```python
from build123d import *

# Parameters (mm, degrees)
F0_R      = 16.5
F17_DEPTH = 12
F18_DEPTH = 2


with BuildPart() as f17:
    # F0 (on Top) → F17 (new body)
    with BuildSketch(Plane.XY):
        with BuildLine():
            ThreePointArc((18.917614, -8.685167), (19.797247, -6.432516), (20.409685, -4.093046))
            ThreePointArc((20.409685, -4.093046), (20.714215, -2.056585), (20.816058, 0))
            ThreePointArc((20.816058, 0), (20.489002, 3.675464), (19.518114, 7.235432))
            ThreePointArc((19.518114, 7.235432), (18.547243, 9.450292), (17.326047, 11.537605))
            ThreePointArc((17.326047, 11.537605), (13.518948, 15.828654), (8.685167, 18.917614))
            ThreePointArc((8.685167, 18.917614), (6.432516, 19.797247), (4.093046, 20.409685))
            ThreePointArc((4.093046, 20.409685), (-1.633209, 20.751889), (-7.235432, 19.518114))
            ThreePointArc((-7.235432, 19.518114), (-9.450292, 18.547243), (-11.537605, 17.326047))
            ThreePointArc((-11.537605, 17.326047), (-15.828654, 13.518948), (-18.917614, 8.685167))
            ThreePointArc((-18.917614, 8.685167), (-19.797247, 6.432516), (-20.409685, 4.093046))
            ThreePointArc((-20.409685, 4.093046), (-20.751889, -1.633209), (-19.518114, -7.235432))
            ThreePointArc((-19.518114, -7.235432), (-18.547243, -9.450292), (-17.326047, -11.537605))
            ThreePointArc((-17.326047, -11.537605), (-13.518948, -15.828654), (-8.685167, -18.917614))
            ThreePointArc((-8.685167, -18.917614), (-6.432516, -19.797247), (-4.093046, -20.409685))
            ThreePointArc((-4.093046, -20.409685), (1.633209, -20.751889), (7.235432, -19.518114))
            ThreePointArc((7.235432, -19.518114), (9.450292, -18.547243), (11.537605, -17.326047))
            ThreePointArc((11.537605, -17.326047), (15.828654, -13.518948), (18.917614, -8.685167))
        make_face()
        Circle(F0_R, mode=Mode.SUBTRACT)
        with BuildLine():
            ThreePointArc((4.093046, 20.409685), (6.432516, 19.797247), (8.685167, 18.917614))
            Line((8.685167, 18.917614), (11.775337, 28.428179))
            Line((11.775337, 28.428179), (7.183216, 29.92025))
            Line((7.183216, 29.92025), (4.093046, 20.409685))
        make_face()
        Polygon((11.775337, 28.428179), (16.07751, 26.236113), (20.629834, 29.030011), (15.834552, 31.89982), (10.649371, 33.98415), (7.183216, 29.92025), align=None)
        Polygon((-16.07751, 26.236113), (-11.775337, 28.428179), (-7.183216, 29.92025), (-5.939822, 35.114813), (-11.35986, 33.753298), (-16.50018, 31.560666), align=None)
        with BuildLine():
            ThreePointArc((-11.537605, 17.326047), (-9.450292, 18.547243), (-7.235432, 19.518114))
            Line((-7.235432, 19.518114), (-11.775337, 28.428179))
            Line((-11.775337, 28.428179), (-16.07751, 26.236113))
            Line((-16.07751, 26.236113), (-11.537605, 17.326047))
        make_face()
        Polygon((-29.92025, 7.183216), (-28.428179, 11.775337), (-26.236113, 16.07751), (-29.030011, 20.629834), (-31.89982, 15.834552), (-33.98415, 10.649371), align=None)
        with BuildLine():
            ThreePointArc((-20.409685, 4.093046), (-19.797247, 6.432516), (-18.917614, 8.685167))
            Line((-18.917614, 8.685167), (-28.428179, 11.775337))
            Line((-28.428179, 11.775337), (-29.92025, 7.183216))
            Line((-29.92025, 7.183216), (-20.409685, 4.093046))
        make_face()
        Polygon((-31.560666, -16.50018), (-26.236113, -16.07751), (-28.428179, -11.775337), (-29.92025, -7.183216), (-35.114813, -5.939822), (-33.753298, -11.35986), align=None)
        with BuildLine():
            Line((-26.236113, -16.07751), (-17.326047, -11.537605))
            ThreePointArc((-17.326047, -11.537605), (-18.547243, -9.450292), (-19.518114, -7.235432))
            Line((-19.518114, -7.235432), (-28.428179, -11.775337))
            Line((-28.428179, -11.775337), (-26.236113, -16.07751))
        make_face()
        Polygon((-10.649371, -33.98415), (-7.183216, -29.92025), (-11.775337, -28.428179), (-16.07751, -26.236113), (-20.629834, -29.030011), (-15.834552, -31.89982), align=None)
        with BuildLine():
            Line((-7.183216, -29.92025), (-4.093046, -20.409685))
            ThreePointArc((-4.093046, -20.409685), (-6.432516, -19.797247), (-8.685167, -18.917614))
            Line((-8.685167, -18.917614), (-11.775337, -28.428179))
            Line((-11.775337, -28.428179), (-7.183216, -29.92025))
        make_face()
        Polygon((16.50018, -31.560666), (16.07751, -26.236113), (11.775337, -28.428179), (7.183216, -29.92025), (5.939822, -35.114813), (11.35986, -33.753298), align=None)
        with BuildLine():
            Line((16.07751, -26.236113), (11.537605, -17.326047))
            ThreePointArc((11.537605, -17.326047), (9.450292, -18.547243), (7.235432, -19.518114))
            Line((7.235432, -19.518114), (11.775337, -28.428179))
            Line((11.775337, -28.428179), (16.07751, -26.236113))
        make_face()
        Polygon((33.98415, -10.649371), (29.92025, -7.183216), (28.428179, -11.775337), (26.236113, -16.07751), (29.030011, -20.629834), (31.89982, -15.834552), align=None)
        with BuildLine():
            Line((28.428179, -11.775337), (29.92025, -7.183216))
            Line((29.92025, -7.183216), (20.409685, -4.093046))
            ThreePointArc((20.409685, -4.093046), (19.797247, -6.432516), (18.917614, -8.685167))
            Line((18.917614, -8.685167), (28.428179, -11.775337))
        make_face()
        Polygon((28.428179, 11.775337), (29.92025, 7.183216), (35.114813, 5.939822), (33.753298, 11.35986), (31.560666, 16.50018), (26.236113, 16.07751), align=None)
        with BuildLine():
            Line((19.518114, 7.235432), (28.428179, 11.775337))
            Line((28.428179, 11.775337), (26.236113, 16.07751))
            Line((26.236113, 16.07751), (17.326047, 11.537605))
            ThreePointArc((17.326047, 11.537605), (18.547243, 9.450292), (19.518114, 7.235432))
        make_face()
    extrude(amount=F17_DEPTH)

    # F9 (on face) + F10 (on face) + F11 (on face) + F7 (on face) + F8 (on face) + F1 (on face) + F2 (on face) + F16 (on face) + F15 (on face) + F3 (on face) + F14 (on face) + F4 (on face) + F13 (on face) + F5 (on face) + F12 (on face) + F6 (on face) → F18 (join)
    with BuildSketch(Plane.XY):
        Polygon((-23.398026, 19.983802), (-19.983802, 23.398026), (-16.07751, 26.236113), (-16.50018, 31.560666), (-21.234212, 28.590905), (-25.445386, 24.917141), (-29.030011, 20.629834), (-26.236113, 16.07751), align=None)
    with BuildSketch(Plane.XY):
        Polygon((-2.414221, 30.675584), (2.414221, 30.675584), (7.183216, 29.92025), (10.649371, 33.98415), (5.201968, 35.231677), (-0.373526, 35.611684), (-5.939822, 35.114813), (-7.183216, 29.92025), align=None)
    with BuildSketch(Plane.XY):
        Polygon((19.983802, 23.398026), (23.398026, 19.983802), (26.236113, 16.07751), (31.560666, 16.50018), (28.590905, 21.234212), (24.917141, 25.445386), (20.629834, 29.030011), (16.07751, 26.236113), align=None)
    with BuildSketch(Plane.XY):
        with BuildLine():
            ThreePointArc((8.685167, 18.917614), (13.518948, 15.828654), (17.326047, 11.537605))
            Line((17.326047, 11.537605), (26.236113, 16.07751))
            Line((26.236113, 16.07751), (23.398026, 19.983802))
            Line((23.398026, 19.983802), (19.983802, 23.398026))
            Line((19.983802, 23.398026), (16.07751, 26.236113))
            Line((16.07751, 26.236113), (11.775337, 28.428179))
            Line((11.775337, 28.428179), (8.685167, 18.917614))
        make_face()
    with BuildSketch(Plane.XY):
        with BuildLine():
            Line((-11.775337, 28.428179), (-7.235432, 19.518114))
            ThreePointArc((-7.235432, 19.518114), (-1.633209, 20.751889), (4.093046, 20.409685))
            Line((4.093046, 20.409685), (7.183216, 29.92025))
            Line((7.183216, 29.92025), (2.414221, 30.675584))
            Line((2.414221, 30.675584), (-2.414221, 30.675584))
            Line((-2.414221, 30.675584), (-7.183216, 29.92025))
            Line((-7.183216, 29.92025), (-11.775337, 28.428179))
        make_face()
    with BuildSketch(Plane.XY):
        with BuildLine():
            Line((-28.428179, 11.775337), (-18.917614, 8.685167))
            ThreePointArc((-18.917614, 8.685167), (-15.828654, 13.518948), (-11.537605, 17.326047))
            Line((-11.537605, 17.326047), (-16.07751, 26.236113))
            Line((-16.07751, 26.236113), (-19.983802, 23.398026))
            Line((-19.983802, 23.398026), (-23.398026, 19.983802))
            Line((-23.398026, 19.983802), (-26.236113, 16.07751))
            Line((-26.236113, 16.07751), (-28.428179, 11.775337))
        make_face()
    with BuildSketch(Plane.XY):
        with BuildLine():
            Line((-29.92025, -7.183216), (-28.428179, -11.775337))
            Line((-28.428179, -11.775337), (-19.518114, -7.235432))
            ThreePointArc((-19.518114, -7.235432), (-20.751889, -1.633209), (-20.409685, 4.093046))
            Line((-20.409685, 4.093046), (-29.92025, 7.183216))
            Line((-29.92025, 7.183216), (-30.675584, 2.414221))
            Line((-30.675584, 2.414221), (-30.675584, -2.414221))
            Line((-30.675584, -2.414221), (-29.92025, -7.183216))
        make_face()
    with BuildSketch(Plane.XY):
        Polygon((-30.675584, -2.414221), (-30.675584, 2.414221), (-29.92025, 7.183216), (-33.98415, 10.649371), (-35.231677, 5.201968), (-35.611684, -0.373526), (-35.114813, -5.939822), (-29.92025, -7.183216), align=None)
    with BuildSketch(Plane.XY):
        Polygon((-19.983802, -23.398026), (-23.398026, -19.983802), (-26.236113, -16.07751), (-31.560666, -16.50018), (-28.590905, -21.234212), (-24.917141, -25.445386), (-20.629834, -29.030011), (-16.07751, -26.236113), align=None)
    with BuildSketch(Plane.XY):
        with BuildLine():
            Line((-16.07751, -26.236113), (-11.775337, -28.428179))
            Line((-11.775337, -28.428179), (-8.685167, -18.917614))
            ThreePointArc((-8.685167, -18.917614), (-13.518948, -15.828654), (-17.326047, -11.537605))
            Line((-17.326047, -11.537605), (-26.236113, -16.07751))
            Line((-26.236113, -16.07751), (-23.398026, -19.983802))
            Line((-23.398026, -19.983802), (-19.983802, -23.398026))
            Line((-19.983802, -23.398026), (-16.07751, -26.236113))
        make_face()
    with BuildSketch(Plane.XY):
        Polygon((2.414221, -30.675584), (-2.414221, -30.675584), (-7.183216, -29.92025), (-10.649371, -33.98415), (-5.201968, -35.231677), (0.373526, -35.611684), (5.939822, -35.114813), (7.183216, -29.92025), align=None)
    with BuildSketch(Plane.XY):
        with BuildLine():
            Line((7.183216, -29.92025), (11.775337, -28.428179))
            Line((11.775337, -28.428179), (7.235432, -19.518114))
            ThreePointArc((7.235432, -19.518114), (1.633209, -20.751889), (-4.093046, -20.409685))
            Line((-4.093046, -20.409685), (-7.183216, -29.92025))
            Line((-7.183216, -29.92025), (-2.414221, -30.675584))
            Line((-2.414221, -30.675584), (2.414221, -30.675584))
            Line((2.414221, -30.675584), (7.183216, -29.92025))
        make_face()
    with BuildSketch(Plane.XY):
        Polygon((25.445386, -24.917141), (29.030011, -20.629834), (26.236113, -16.07751), (23.398026, -19.983802), (19.983802, -23.398026), (16.07751, -26.236113), (16.50018, -31.560666), (21.234212, -28.590905), align=None)
    with BuildSketch(Plane.XY):
        with BuildLine():
            Line((23.398026, -19.983802), (26.236113, -16.07751))
            Line((26.236113, -16.07751), (28.428179, -11.775337))
            Line((28.428179, -11.775337), (18.917614, -8.685167))
            ThreePointArc((18.917614, -8.685167), (15.828654, -13.518948), (11.537605, -17.326047))
            Line((11.537605, -17.326047), (16.07751, -26.236113))
            Line((16.07751, -26.236113), (19.983802, -23.398026))
            Line((19.983802, -23.398026), (23.398026, -19.983802))
        make_face()
    with BuildSketch(Plane.XY):
        Polygon((35.114813, 5.939822), (29.92025, 7.183216), (30.675584, 2.414221), (30.675584, -2.414221), (29.92025, -7.183216), (33.98415, -10.649371), (35.231677, -5.201968), (35.611684, 0.373526), align=None)
    with BuildSketch(Plane.XY):
        with BuildLine():
            Line((29.92025, -7.183216), (30.675584, -2.414221))
            Line((30.675584, -2.414221), (30.675584, 2.414221))
            Line((30.675584, 2.414221), (29.92025, 7.183216))
            Line((29.92025, 7.183216), (28.428179, 11.775337))
            Line((28.428179, 11.775337), (19.518114, 7.235432))
            ThreePointArc((19.518114, 7.235432), (20.489002, 3.675464), (20.816058, 0))
            ThreePointArc((20.816058, 0), (20.714215, -2.056585), (20.409685, -4.093046))
            Line((20.409685, -4.093046), (29.92025, -7.183216))
        make_face()
    extrude(amount=F18_DEPTH)


solid = f17.part
```
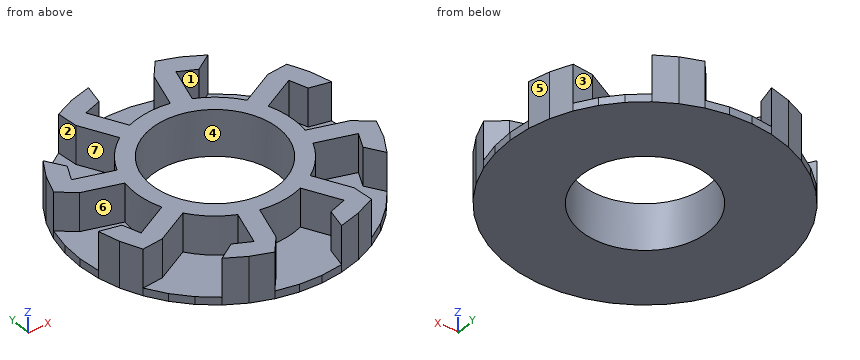
The listing builds one solid part. Answer for the finished solid, in the listing's coordinates (mm). Face numbers are marked on the shaded views. A direction names the side the tool comes from. Coordinates: 2 decimals unless noted, no trailing zeros. Loops run counter-clockwise (first coordinate to the right, second up) from the corner with the lowest first, then second, coordinate; pieces in that order, holes last. Notation, with made-up numbers: M 67.5,-34 L 118.5,-34 A4 cw 118.5,-30 Z; hole C 81.25,-19 d3. An arc over 180 degrees is marked long. Answer as CSV lines item,"result". Start each with the question number.
(1) Find the intervals of material crossed by L1, parallel to Y at x = 0, z = 9.5; L2, parallel to Y at x = -27.5, z = 10; L3, parallel to X at y = 15, z = 10, in increasing order. Write a range as [from, to].
(2) The part is cut by section A-A (y = 15). Give the vertices of the cut face in (x, z), and give its area (3 significant figures).
(3) Given pin 1 (5 mm diameter, centred on x = 16.5, y = -18.5, fed in from +Z); pin 2 (6 mm diameter, centred on x = 22.5, z = 10.5, fed in from +Y); pin 3 (4 mm diameter, centred on y = -18.5, z = 2, fed in from -X), each flat-ended and moving along its own axis, determine where each tip first touches the part or whether it passes through.
(4) For the marked faces 1, 2 and 3, determine the directions among +Z, -Z, +X, -X, +Y, -Y from which every point of the face is accessible in a straight line to the end or side of a thin tool.
(5) The mould has two halves that part along X. Classify the marked faces 4, 5, 6 and 7: pulls with the +X half, pulls with the -X half, needs draft (parallel to the pull), parting line crosses it, or undercut.
Determined:
1,L1,"[-20.82, -16.5], [16.5, 20.82]"
1,L2,"[-16.18, -11.3], [6.4, 11.47], [13.6, 18.14]"
1,L3,"[-32.24, -26.79], [-14.43, -6.87], [6.87, 14.43], [24.12, 32.2]"
2,outline,"M -32.24,0 L -6.87,0 L -6.87,12 L -14.43,12 L -14.43,2 L -26.79,2 L -26.79,12 L -32.24,12 Z; M 6.87,0 L 32.2,0 L 32.2,12 L 24.12,12 L 24.12,2 L 14.43,2 L 14.43,12 L 6.87,12 Z"
2,area,"388 mm2"
3,pin 1,"z = 2"
3,pin 2,"y = 29.71"
3,pin 3,"x = -31.56"
4,face 1,"+Z"
4,face 2,"+Z, -X"
4,face 3,"+Z, +Y"
5,face 4,"undercut"
5,face 5,"pulls with the +X half"
5,face 6,"pulls with the -X half"
5,face 7,"undercut"
